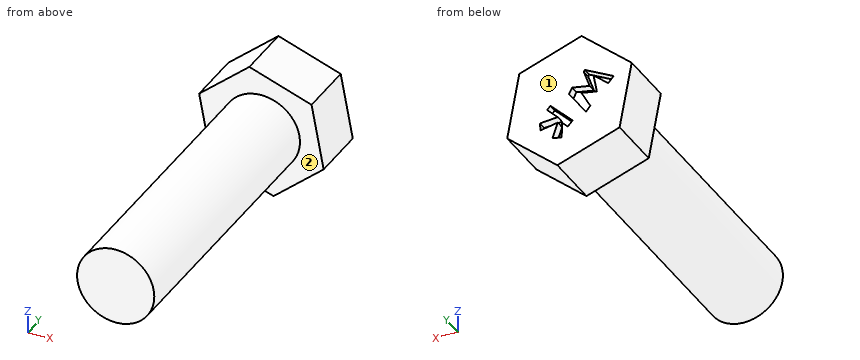
Autodesk Inventor part; units mm, degrees
ref_plane "YZ Plane" through (0, 0, 0) normal (1, 0, 0) x (0, 1, 0)
ref_plane "XZ Plane" through (0, 0, 0) normal (0, 1, 0) x (-1, 0, 0)
ref_plane "XY Plane" through (0, 0, 0) normal (0, 0, 1) x (1, 0, 0)
sketch "Sketch1" plane through (0, 0, 0) normal (0, 0, 1) x (1, 0, 0)
  line L0 (-2.7545, 0) -> (0.6745, 0)
  line L1 (0.6745, 0) -> (0.6745, 25.4)
  line L2 (0.6745, 25.4) -> (-2.7545, 25.4)
  line L3 (-2.7545, 25.4) -> (-2.7545, 0)
  point P0 (0, 0)
  dimension "d0" = 3.429
  dimension "d1" = 25.4
revolve "Revolution1" add sketch "Sketch1" angle 360 about axis through (-2.7545, 25.4, 0) along (0, -1, 0)
sketch "Sketch2" plane through (-2.7545, 25.4, 0) normal (0, 1, 0) x (1, 0, 0)
  circle A0 centre (0, 0) radius 3.429
  line L0 (-1.0753, -5.7665) -> (-5.5316, -1.952)
  line L1 (-5.5316, -1.952) -> (-4.4562, 3.8145)
  line L2 (-4.4562, 3.8145) -> (1.0753, 5.7665)
  line L3 (1.0753, 5.7665) -> (5.5316, 1.952)
  line L4 (5.5316, 1.952) -> (4.4562, -3.8145)
  line L5 (4.4562, -3.8145) -> (-1.0753, -5.7665)
  point P0 (2.7545, 0)
  dimension "d3" = 5.08
extrude "Extrusion1" add sketch "Sketch2" along normal blind 5.08 contours A0 | L0 L1 L2 L3 L4 L5
thread "Thread1"
sketch "Sketch3" plane through (-2.7545, 30.48, 0) normal (0, 1, 0) x (1, 0, 0)
  line L0 (5.5316, 1.952) -> (4.4562, -3.8145)
  line L1 (1.0753, 5.7665) -> (5.5316, 1.952)
  line L2 (-4.4562, 3.8145) -> (1.0753, 5.7665)
  line L3 (-3.9194, -1.1734) -> (-1.366, -2.4875)
  line L4 (-1.366, -2.4875) -> (-1.2813, -2.3228)
  line L5 (-1.2813, -2.3228) -> (-1.7974, -0.8601)
  line L6 (-1.7974, -0.8601) -> (-0.2306, -1.1523)
  line L7 (-0.2306, -1.1523) -> (0.0392, -0.6281)
  line L8 (0.0392, -0.6281) -> (-1.4654, 1.4765)
  line L9 (-1.4654, 1.4765) -> (-1.8516, 1.0253)
  line L10 (-1.8516, 1.0253) -> (-1.0682, -0.4113)
  line L11 (-1.0682, -0.4113) -> (-2.4324, -0.1569)
  line L12 (-2.4324, -0.1569) -> (-2.1392, -1.7523)
  line L13 (-2.1392, -1.7523) -> (-3.4526, -0.6281)
  line L14 (-3.4526, -0.6281) -> (-3.9194, -1.1734)
  line L15 (-0.2889, 1.952) -> (1.6905, 0)
  line L16 (1.6905, 0) -> (1.9932, 0.307)
  line L17 (1.9932, 0.307) -> (1.0361, 1.2509)
  line L18 (1.0361, 1.2509) -> (2.6233, 1.3796)
  line L19 (2.6233, 1.3796) -> (2.569, 2.0493)
  line L20 (2.569, 2.0493) -> (1.0361, 1.7676)
  line L21 (1.0361, 1.7676) -> (1.5146, 3.1041)
  line L22 (1.5146, 3.1041) -> (0.7008, 3.2559)
  line L23 (0.7008, 3.2559) -> (0.6427, 1.9085)
  line L24 (0.6427, 1.9085) -> (0.1487, 2.3957)
  line L25 (0.1487, 2.3957) -> (-0.2889, 1.952)
  point P0 (2.7545, 0)
extrude "Extrusion2" cut sketch "Sketch3" against normal blind 0.762
properties part number "1in bolt"
Verification items for the finished model (mm, model axes). Face numbers are marked on the shaded views. A direction names the side the tool comes from. Coordinates: 2 decimals unless noted, no trailing zeros. Order: outer loops, then holes, each group sorted by start corner. A loop starts at its lowest first (then second) coordinate and runs counter-clockwise, first axis right, second up. Notation, with made-up numbers: M 85,39 L 122,39 A30 cw 122,65 Z; hole C 36,7.5 d9. An arc over 180 degrees is marked long. One line per item, written item: value. Start each with the question number.
Item 1: Access from +Z, -Z, +X, -X, +Y, -Y to the whole of each face (thin tool, end or side, straight path). Record for the marked faces 1 and 2.
Item 2: Sectioned sample at B-B (x = 2). Enter the section's corners in (y, z), then the cut area to 3 significant figures.
Item 3: Gauge pin test, flat ends, axial feed: pin 1 (4 mm diameter, centred on x = -7, z = -4, fed in from -Y); pin 2 (4 mm diameter, centred on x = -2.5, y = 17, fed in from +Z); pin 3 (1 mm diameter, centred on y = 10, z = 2.5, fed in from -X); pin 4 (4 mm diameter, centred on x = -6, z = 4, fed in from +Y). Record the tip position at first contact, or that the pin passes through.
Item 4: Scan lines: probe 1 along Y at (x, z) = (-0.25, 2.5); probe 2 along Y at (x, z) = (-3.25, 0); probe 3 along X at (y, z) = (20, 2.25). Record each from-to range of solid material in increasing order.
Item 5: Sectioned sample at A-A (y = 23.5). Enter the section's corners in (x, z), then the cut area to 3 significant figures.
Conclusion:
1. face 1: +Z, -Z, +X, -X, +Y
1. face 2: -Y
2. outline: M 25.4,-2.62 L 30.48,-2.62 L 30.48,2.21 L 25.4,2.21 Z
2. area: 24.5 mm^2
3. pin 1: stops at y = 25.4
3. pin 2: stops at z = 3.43
3. pin 3: stops at x = -5.54
3. pin 4: stops at y = 30.48
4. probe 1: y = 25.4 to 30.48
4. probe 2: y = 0 to 29.72
4. probe 3: x = -5.34 to -0.17
5. outline: C -2.75,0 d6.86
5. area: 36.9 mm^2
